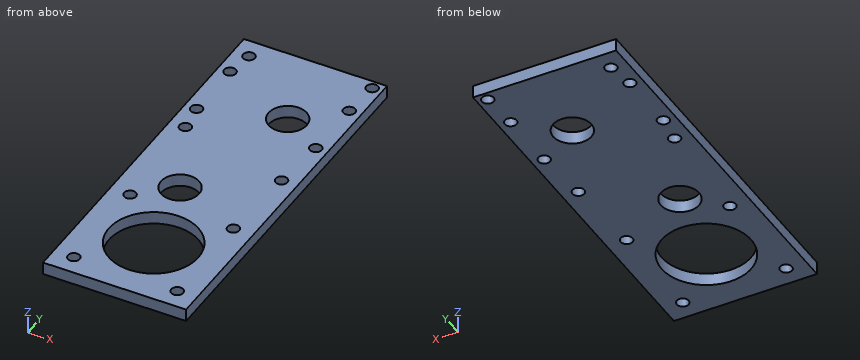
```python
from build123d import *

# Parameters (mm, degrees)
SKETCH2_W           = 36
SKETCH2_H           = 93
SKETCH2_R           = 1.5
SKETCH2_R_2         = 11.25
SKETCH2_R_3         = 4.8
BOSS_EXTRUDE1_DEPTH = 3.175
SKETCH3_R           = 1.5
CUT_EXTRUDE1_DEPTH  = 16


with BuildPart() as part:
    # Sketch2 → Boss-Extrude1 (new body)
    with BuildSketch(Plane.XY):
        with Locations((0, 7.942942894)):
            Rectangle(SKETCH2_W, SKETCH2_H)
        with Locations((13.053786058, -33.557057106)):
            Circle(SKETCH2_R, mode=Mode.SUBTRACT)
        with Locations((13.053786058, -7.557057106)):
            Circle(SKETCH2_R, mode=Mode.SUBTRACT)
        with Locations((-12.946213942, -33.557057106)):
            Circle(SKETCH2_R, mode=Mode.SUBTRACT)
        with Locations((-12.946213942, -7.557057106)):
            Circle(SKETCH2_R, mode=Mode.SUBTRACT)
        with Locations((0.053786058, -20.557057106)):
            Circle(SKETCH2_R_2, mode=Mode.SUBTRACT)
        with Locations((-4.475, 0)):
            Circle(SKETCH2_R_3, mode=Mode.SUBTRACT)
        with Locations((4.475, 33.370645783)):
            Circle(SKETCH2_R_3, mode=Mode.SUBTRACT)
        with Locations((14, 13)):
            Circle(SKETCH2_R, mode=Mode.SUBTRACT)
        with Locations((-14, 20)):
            Circle(SKETCH2_R, mode=Mode.SUBTRACT)
        with Locations((-14, 49.442942894)):
            Circle(SKETCH2_R, mode=Mode.SUBTRACT)
        with Locations((15.5, 52.187088466)):
            Circle(SKETCH2_R, mode=Mode.SUBTRACT)
    extrude(amount=BOSS_EXTRUDE1_DEPTH)

    # Sketch3 → Cut-Extrude1 (cut)
    with BuildSketch(Plane.XY.offset(3.175)):
        with Locations((-15, 42.5)):
            Circle(SKETCH3_R)
        with Locations((15, 42.5)):
            Circle(SKETCH3_R)
        with Locations((-15, 27)):
            Circle(SKETCH3_R)
        with Locations((15, 27)):
            Circle(SKETCH3_R)
    extrude(amount=-CUT_EXTRUDE1_DEPTH, mode=Mode.SUBTRACT)


solid = part.part
```
Source: CAD feature listing. Evaluate the final solid. Frame: model axes, mm. Round coordinates to 2 decimals unless told otherwise and drop trailing zeros. Loops run counter-clockwise (first coordinate to the right, second up) from the corner with the lowest first, then second, coordinate; pieces in that order, holes last. Notation, with made-up numbers: M 47,21 L 101,21 A29 ccw 101,51 Z; hole C 85,-28 d2. An arc over 180 degrees is marked long. Use a Markdown table: item, result. Add a question column.
1. Section query B-B on z = 2. Give the number of separate pieces and of enclosed holes in the cut face, then the cut area to 3 significant figures.
2. Section query A-A on y = 20. Return the cut outline in (x, z) (3 decimals).
3. Section query C-C on x = -7.5. Return the cut outline in (y, z) (3 decimals).
4. Section query D-D on y = 0. Return the cut outline in (x, z) (3 decimals), then the cut area to 3 significant figures.
5. Line query: line 1 (Y direction, x = -3.5, z = 2.4); line 2 (Y direction, x = -15, z = 0.75); line 3 (X direction, y = 33.5, z = 2.05). Output: solid intervals per line, ascending.
Reported:
| question | item | result |
|---|---|---|
| 1 | separate pieces | 1 |
| 1 | enclosed holes | 15 |
| 1 | area | 2,720 mm² |
| 2 | outline | M -18,0 L -15.5,0 L -15.5,3.175 L -18,3.175 Z; M -12.5,0 L 18,0 L 18,3.175 L -12.5,3.175 Z |
| 3 | outline | M -38.557,0 L -28.894,0 L -28.894,3.175 L -38.557,3.175 Z; M -12.22,0 L -3.727,0 L -3.727,3.175 L -12.22,3.175 Z; M 3.727,0 L 54.443,0 L 54.443,3.175 L 3.727,3.175 Z |
| 4 | outline | M -18,0 L -9.275,0 L -9.275,3.175 L -18,3.175 Z; M 0.325,0 L 18,0 L 18,3.175 L 0.325,3.175 Z |
| 4 | area | 83.8 mm² |
| 5 | line 1 | y = -38.56 to -31.23, -9.88 to -4.7, 4.7 to 54.44 |
| 5 | line 2 | y = -38.56 to 18.88, 21.12 to 25.5, 28.5 to 41, 44 to 48.32, 50.56 to 54.44 |
| 5 | line 3 | x = -18 to -0.32, 9.27 to 18 |
